```python
from build123d import *

# Parameters (mm, degrees)
BOSS_EXTRUDE1_DEPTH = 3
SKETCH2_R           = 4.3
BOSS_EXTRUDE2_DEPTH = 8
SKETCH3_R           = 2
BOSS_EXTRUDE3_DEPTH = 4


with BuildPart() as part:
    # Sketch1 → Boss-Extrude1 (new body)
    with BuildSketch(Plane(origin=(0, 0, 0), x_dir=(1, 0, 0), z_dir=(0, 1, 0))):
        Polygon((0, -4.618802154), (4, -2.309401077), (4, 2.309401077), (0, 4.618802154), (-4, 2.309401077), (-4, -2.309401077), align=None)
    extrude(amount=BOSS_EXTRUDE1_DEPTH)

    # Sketch2 → Boss-Extrude2 (add)
    with BuildSketch(Plane.XZ):
        Circle(SKETCH2_R)
    extrude(amount=BOSS_EXTRUDE2_DEPTH)

    # Sketch3 → Boss-Extrude3 (add)
    with BuildSketch(Plane(origin=(0, 3, 0), x_dir=(1, 0, 0), z_dir=(0, 1, 0))):
        Circle(SKETCH3_R)
    extrude(amount=BOSS_EXTRUDE3_DEPTH)


solid = part.part
```
For this review, take the finished solid that the model builds, in its own axes (mm). A direction names the side the tool comes from. Coordinates: 2 decimals unless noted, no trailing zeros. Loops run counter-clockwise (first coordinate to the right, second up) from the corner with the lowest first, then second, coordinate; pieces in that order, holes last. Notation, with made-up numbers: (-5.5, 32.5) - (30.5, 32.5) arc R20 cw to (30.5, 64.5) - close; hole circle Ø9 at (50, 58.25). An arc over 180 degrees is marked (long way). Use one line per item in the form item = value. Start each with the question number.
1) Take a section at B-B (x = -1.5). State the section outline as (y, z) points, plus the area to 3 significant figures.
2) Take a section at D-D (z = -2.5). State the section outline as (x, y) points, plus the area to 3 significant figures.
3) For pin 1 (0.8 mm diameter, centred on x = -2.5, z = -3.5, fed in from +Y); pin 2 (3 mm diameter, centred on x = -0.5, y = -4.5, fed in from -Z); pin 3 (0.5 mm diameter, centred on x = 2.5, z = 3.5, fed in from +Y), all flat-tipped, find the tip position at first contact; note any pin that passes through.
4) Take a section at C-C (y = 3.25). State the section outline as (x, z) points, plus the area to 3 significant figures.
5) Take a section at A-A (z = 0.5). State the section outline as (x, y) points.
6) For faces 1 (the face through (-1.97, 1.48, -3.48)), 2 (the face through (-4, 1, 0)), 3 (the face through (-4.296, -3.944, 0.189)), list the 3-axis set-ups (+Z, -Z, +X, -X, +Y, -Y) from which the entire face can be reached by the end or side of a thin tool; tool diameter is ignored.
7) To check wall thickness, follow probe 1 along Y at (x, z) = (0.25, 2.25); probe 2 along X at (y, z) = (5.75, 0); probe 3 along Z at (x, y) = (-3, -1). State the ranges of each line that lie inside material, in increasing order. Write a range as from..to.
From the geometry:
q1.outline = (-8, -4.03) - (0, -4.03) - (0, -3.75) - (3, -3.75) - (3, -1.32) - (7, -1.32) - (7, 1.32) - (3, 1.32) - (3, 3.75) - (0, 3.75) - (0, 4.03) - (-8, 4.03) - close
q1.area = 97.6 mm2
q2.outline = (-3.67, 0) - (-3.5, 0) - (-3.5, -8) - (3.5, -8) - (3.5, 0) - (3.67, 0) - (3.67, 3) - (-3.67, 3) - close
q2.area = 78.0 mm2
q3.pin_1 = 3
q3.pin_2 = -4.3
q3.pin_3 = 0
q4.outline = circle Ø4 at (0, 0)
q4.area = 12.6 mm2
q5.outline = (-4.27, -8) - (4.27, -8) - (4.27, 0) - (4, 0) - (4, 3) - (1.94, 3) - (1.94, 7) - (-1.94, 7) - (-1.94, 3) - (-4, 3) - (-4, 0) - (-4.27, 0) - close
q6.face_1 = -Z, -X, +Y
q6.face_2 = +Z, -Z, -X, +Y
q6.face_3 = -Y
q7.probe_1 = -8..3
q7.probe_2 = -2..2
q7.probe_3 = -3.08..3.08
